For this review, take the finished solid that the model builds, in its own axes (mm). A direction names the side the tool comes from. Round coordinates to 2 decimals unless told otherwise and drop trailing zeros. Write each loop counter-clockwise with the first axis right and the second up, starting at its lowest first coordinate (ties: lowest second). Pieces come first, ordered by that corner, then holes. Notation, with made-up numbers: (23, 3) - (52, 3) arc R10 cw to (52, 7) - close; hole circle Ø1 at (62, 63). An arc over 180 degrees is marked (long way). One line per item, written item: value. Start each with the question number.
Q1. Add section A-A on z = 9. Write out the cut boundary in (x, y).
Q2. Add section B-B on x = 40. Write out the cut boundary in (y, z).
Q3. Add section C-C on x = 144.5. Write out the cut boundary in (y, z).
Q4. Tool access review of faces 4 (the face through (74, 0, 9)), 5 (the face through (50, 7, 9)), 6 (the face through (137.675, 2.535, -6.084)), 7 (the face through (153, 13.25, -26)), 8 (the face through (152.465, -4.049, -33.126)): name each direction out of +Z, -Z, +X, -X, +Y, -Y from which nothing blocks a thin tool from reaching the whole face with its end or side.
Q5. Clearance check with flat-ended pins moving along their axes: pin 1 Ø1.5 at (x, y) = (153.5, 17.5) entering from +Z; pin 2 Ø2 at (y, z) = (-1, -28) entering from -X; pin 3 Ø15 at (x, z) = (79.5, -2.5) entering from +Y. State where each tip first meets the part, or that it passes through.
Q6. Add section D-D on y = 19.5. Write out the cut boundary in (x, z), and give its area (3 significant figures).
Q7. For probe 1 along X at (y, z) = (2, 9); probe 2 along Y at (x, z) = (151, -18); probe 3 along X at (y, z) = (5.5, -22.5), list the stretches that pass through material, from the lowest coordinate up.
Q8. Mouldability with a two-part tool opening along Y and no side actions: class faces 1 (the face through (152, -5, 3)), 2 (the face through (152, -14, -12)), 3 (the face through (152.54, 14.96, -16.25)) as +Y half, -Y half, draft (parallel to the pull), parting line (faces both ways), or undercut.
```python
from build123d import *

# Parameters (mm, degrees)
SKETCH_1_W          = 150
SKETCH_1_H          = 18
EXTRUDE_1_DEPTH     = 5
SKETCH_2_R          = 2.5
CUT_EXTRUDE_1_DEPTH = 152.158856836
EXTRUDE_3_DEPTH     = 5
CUT_EXTRUDE_2_REACH = 164.158
SKETCH_8_R          = 1.75
EXTRUDE_4_DEPTH     = 100
EXTRUDE_5_DEPTH     = 5


with BuildPart() as part:
    # 草图1 → 凸台-拉伸1 (new body)
    with BuildSketch(Plane(origin=(0, 0, 0), x_dir=(1, 0, 0), z_dir=(0, 1, 0))):
        with Locations((75, -9)):
            Rectangle(SKETCH_1_W, SKETCH_1_H)
    extrude(amount=EXTRUDE_1_DEPTH)

    # 草图2 → 切除-拉伸1 (cut, through all)
    with BuildSketch(Plane(origin=(0, 5, 0), x_dir=(1, 0, 0), z_dir=(0, 1, 0))):
        with Locations(Location((15, -9, 0), (0, 0, 270))):
            Circle(SKETCH_2_R)
        with Locations(Location((40, -9, 0), (0, 0, 270))):
            Circle(SKETCH_2_R)
    extrude(amount=-CUT_EXTRUDE_1_DEPTH, mode=Mode.SUBTRACT)

    # 草图6 → 凸台-拉伸3 (add)
    with BuildSketch(Plane(origin=(150, 0, 0), x_dir=(0, 0, -1), z_dir=(1, 0, 0))):
        Polygon((12, 15), (12, 22.5), (24, 22.5), (42, 22.5), (42, 9.029805857), (24, -17.5), (12, -17.5), (12, -10), (-18, 0), (-18, 5), align=None)
    extrude(amount=EXTRUDE_3_DEPTH)

    # 草图8 → 切除-拉伸2 (cut, up to next)
    with BuildSketch(Plane(origin=(155, 0, 0), x_dir=(0, 0, -1), z_dir=(1, 0, 0)), mode=Mode.PRIVATE) as cut_extrude_2_sk1:
        with Locations((18, -10)):
            Circle(SKETCH_8_R)
    cut_extrude_2_tool1 = extrude(cut_extrude_2_sk1.sketch, amount=-CUT_EXTRUDE_2_REACH, mode=Mode.PRIVATE) & part.part
    # 草图8 → 切除-拉伸2 (cut, up to next)
    with BuildSketch(Plane(origin=(155, 0, 0), x_dir=(0, 0, -1), z_dir=(1, 0, 0)), mode=Mode.PRIVATE) as cut_extrude_2_sk2:
        with BuildLine():
            Line((18, 16.75), (34, 16.75))
            ThreePointArc((34, 16.75), (35.75, 15), (34, 13.25))
            Line((34, 13.25), (18, 13.25))
            ThreePointArc((18, 13.25), (16.25, 15), (18, 16.75))
        make_face()
    cut_extrude_2_tool2 = extrude(cut_extrude_2_sk2.sketch, amount=-CUT_EXTRUDE_2_REACH, mode=Mode.PRIVATE) & part.part
    add(cut_extrude_2_tool1.solids().sort_by_distance((155, -10, -18))[0], mode=Mode.SUBTRACT)
    add(cut_extrude_2_tool2.solids().sort_by_distance((155, 15, -26))[0], mode=Mode.SUBTRACT)

    # 草图10 → 凸台-拉伸4 (add)
    with BuildSketch(Plane.ZY.offset(-150)):
        Polygon((6, 9), (6, 5), (9, 5), (12, 5), (12, 7), align=None)
    extrude(amount=EXTRUDE_4_DEPTH)

    # 草图11 → 凸台-拉伸5 (add)
    with BuildSketch(Plane(origin=(0, 5, 0), x_dir=(1, 0, 0), z_dir=(0, 1, 0))):
        Polygon((150, 0), (150, 12), (125, 0), align=None)
    extrude(amount=-EXTRUDE_5_DEPTH)


solid = part.part
```
Result set:
1. outline: (0, 0) - (12.5, 0) - (12.5, 5) - (0, 5) - close; (17.5, 0) - (37.5, 0) - (37.5, 5) - (17.5, 5) - close; (42.5, 0) - (150, 0) - (150, -3) - (155, -3) - (155, 8) - (50, 8) - (50, 5) - (42.5, 5) - close
2. outline: (0, 0) - (5, 0) - (5, 6.5) - (0, 6.5) - close; (0, 11.5) - (5, 11.5) - (5, 18) - (0, 18) - close
3. outline: (0, -9.36) - (5, -9.36) - (5, 6) - (9, 6) - (7, 12) - (5, 12) - (5, 18) - (0, 18) - close
4. face 4: +Z, -Z, -X, -Y
4. face 5: +Z, -Z, -X, +Y
4. face 6: -Z, -X, +Y, -Y
4. face 7: +X, -X
4. face 8: -Z, +X, -X, -Y
5. pin 1: stops at z = -12
5. pin 2: stops at x = 150
5. pin 3: stops at y = 5
6. outline: (150, -42) - (155, -42) - (155, -12) - (150, -12) - close
6. area: 150 mm^2
7. probe 1: x = 0 to 12.5, 17.5 to 37.5, 42.5 to 155
7. probe 2: y = -17.5 to -11.75, -8.25 to 13.25, 16.75 to 22.5
7. probe 3: x = 150 to 155
8. face 1: -Y half
8. face 2: draft
8. face 3: undercut
